from build123d import *

# Parameters (mm, degrees)
SKETCH2_W           = 8
SKETCH2_H           = 9
BOSS_EXTRUDE1_DEPTH = 6.8
FILLET1_R           = 1
SKETCH3_W           = 2
SKETCH3_H           = 2
BOSS_EXTRUDE2_DEPTH = 3.2


with BuildPart() as part:
    # Sketch2 → Boss-Extrude1 (new body)
    with BuildSketch(Plane(origin=(0, 0, 0), x_dir=(1, 0, 0), z_dir=(0, 1, 0))):
        with Locations((4, 4.5)):
            Rectangle(SKETCH2_W, SKETCH2_H)
    extrude(amount=BOSS_EXTRUDE1_DEPTH)

    # Fillet1
    fillet1_edges = [part.edges().sort_by_distance(p)[0] for p in [
        (0, 3.4, -9),
        (8, 3.4, -9),
        (8, 3.4, 0),
        (0, 3.4, 0),
    ]]
    fillet(fillet1_edges, radius=FILLET1_R)

    # Sketch3 → Boss-Extrude2 (add)
    with BuildSketch(Plane(origin=(0, 6.8, 0), x_dir=(1, 0, 0), z_dir=(0, 1, 0))):
        with Locations((4, 4.5)):
            Rectangle(SKETCH3_W, SKETCH3_H)
        with BuildLine():
            Line((3, 3.5), (3, 5.5))
            Line((3, 5.5), (2.267949192, 5.5))
            ThreePointArc((2.267949192, 5.5), (2, 4.5), (2.267949192, 3.5))
            Line((2.267949192, 3.5), (3, 3.5))
        make_face()
        with BuildLine():
            Line((3, 5.5), (3, 6.232050808))
            ThreePointArc((3, 6.232050808), (2.585786438, 5.914213562), (2.267949192, 5.5))
            Line((2.267949192, 5.5), (3, 5.5))
        make_face()
        with BuildLine():
            ThreePointArc((5, 6.232050808), (4, 6.5), (3, 6.232050808))
            Line((3, 6.232050808), (3, 5.5))
            Line((3, 5.5), (5, 5.5))
            Line((5, 5.5), (5, 6.232050808))
        make_face()
        with BuildLine():
            Line((5.732050808, 5.5), (5, 5.5))
            Line((5, 5.5), (5, 3.5))
            Line((5, 3.5), (5.732050808, 3.5))
            ThreePointArc((5.732050808, 3.5), (5.931851653, 3.98236191), (6, 4.5))
            ThreePointArc((6, 4.5), (5.931851653, 5.01763809), (5.732050808, 5.5))
        make_face()
        with BuildLine():
            ThreePointArc((5.732050808, 5.5), (5.414213562, 5.914213562), (5, 6.232050808))
            Line((5, 6.232050808), (5, 5.5))
            Line((5, 5.5), (5.732050808, 5.5))
        make_face()
        with BuildLine():
            Line((5, 3.5), (3, 3.5))
            Line((3, 3.5), (3, 2.767949192))
            ThreePointArc((3, 2.767949192), (4, 2.5), (5, 2.767949192))
            Line((5, 2.767949192), (5, 3.5))
        make_face()
        with BuildLine():
            Line((5.732050808, 3.5), (5, 3.5))
            Line((5, 3.5), (5, 2.767949192))
            ThreePointArc((5, 2.767949192), (5.414213562, 3.085786438), (5.732050808, 3.5))
        make_face()
        with BuildLine():
            Line((3, 2.767949192), (3, 3.5))
            Line((3, 3.5), (2.267949192, 3.5))
            ThreePointArc((2.267949192, 3.5), (2.585786438, 3.085786438), (3, 2.767949192))
        make_face()
        with BuildLine():
            ThreePointArc((5, 2.767949192), (4, 2.5), (3, 2.767949192))
            Line((3, 2.767949192), (3, 1.5))
            Line((3, 1.5), (5, 1.5))
            Line((5, 1.5), (5, 2.767949192))
        make_face()
        with BuildLine():
            ThreePointArc((2.267949192, 3.5), (2, 4.5), (2.267949192, 5.5))
            Line((2.267949192, 5.5), (1, 5.5))
            Line((1, 5.5), (1, 3.5))
            Line((1, 3.5), (2.267949192, 3.5))
        make_face()
        with BuildLine():
            Line((5, 7.5), (3, 7.5))
            Line((3, 7.5), (3, 6.232050808))
            ThreePointArc((3, 6.232050808), (4, 6.5), (5, 6.232050808))
            Line((5, 6.232050808), (5, 7.5))
        make_face()
        with BuildLine():
            Line((7, 5.5), (5.732050808, 5.5))
            ThreePointArc((5.732050808, 5.5), (5.931851653, 5.01763809), (6, 4.5))
            ThreePointArc((6, 4.5), (5.931851653, 3.98236191), (5.732050808, 3.5))
            Line((5.732050808, 3.5), (7, 3.5))
            Line((7, 3.5), (7, 5.5))
        make_face()
    extrude(amount=BOSS_EXTRUDE2_DEPTH)


solid = part.part
Verification items for the finished model (mm, model axes). A direction names the side the tool comes from. Give positions to 0.01 mm unless a question says otherwise; leave off trailing zeros. Write each loop counter-clockwise with the first axis right and the second up, starting at its lowest first coordinate (ties: lowest second). Pieces come first, ordered by that corner, then holes. Notation, with made-up numbers: M -9,-25 L -1,-25 A31 ccw -1,7 Z; hole C -18.5,-31.75 d2. An arc over 180 degrees is marked long. Use CSV: the item, a comma, the result in double quotes.
1) Material ranges on line 1 along Y through (x, z) = (4, -8.25); line 2 along X through (y, z) = (7.5, -7); line 3 along X through (y, z) = (8.5, -4), recorded low to high.
Final values:
line 1,"0 to 6.8"
line 2,"3 to 5"
line 3,"1 to 7"
2) Cross-section at A-A (y = 9). Enter the section's corners in (x, z).
Final values:
outline,"M 1,-5.5 L 2.27,-5.5 A2 ccw 3,-6.23 L 3,-7.5 L 5,-7.5 L 5,-6.23 A2 ccw 5.73,-5.5 L 7,-5.5 L 7,-3.5 L 5.73,-3.5 A2 ccw 5,-2.77 L 5,-1.5 L 3,-1.5 L 3,-2.77 A2 ccw 2.27,-3.5 L 1,-3.5 Z"
3) Access from +Z, -Z, +X, -X, +Y, -Y to the whole of each face (thin tool, end or side, straight path). Record for faces 1 (the face through (4, 8, -7.5)), 2 (the face through (6, 8, -3.5)), 3 (the face through (1, 8, -5)).
Final values:
face 1,"-Z, +X, -X, +Y"
face 2,"+Z, +X, +Y"
face 3,"+Z, -Z, -X, +Y"
4) Cross-section at D-D (z = -0.25). Enter the section's corners in (x, y), plus the area to 3 significant figures.
Final values:
outline,"M 0.34,0 L 7.66,0 L 7.66,6.8 L 0.34,6.8 Z"
area,"49.8 mm²"
5) Cross-section at B-B (z = -6.5). Enter the section's corners in (x, y), plus the area to 3 significant figures.
Final values:
outline,"M 0,0 L 8,0 L 8,6.8 L 5,6.8 L 5,10 L 3,10 L 3,6.8 L 0,6.8 Z"
area,"60.8 mm²"
6) Cross-section at C-C (x = 1.5). Enter the section's corners in (y, z).
Final values:
outline,"M 0,-9 L 6.8,-9 L 6.8,-5.5 L 10,-5.5 L 10,-3.5 L 6.8,-3.5 L 6.8,0 L 0,0 Z"
7) Go/stop test with flat-tipped pins: pin 1 Ø1 at (x, y) = (4, 8) entering from -Z; pin 2 Ø1 at (y, z) = (8.5, -4.5) entering from +X; pin 3 Ø0.6 at (x, y) = (2, 8) entering from +Z. Record where each tip stops, or that it passes through.
Final values:
pin 1,"z = -7.5"
pin 2,"x = 7"
pin 3,"z = -3.45"
